from build123d import *


with BuildPart() as part:
    # BodySke → BaseBody (revolve)
    with BuildSketch(Plane.XY, mode=Mode.PRIVATE) as basebody_sk:
        with BuildLine():
            Line((21.808290377, 3.6), (25.5, 3.6))
            Line((25.5, 3.6), (25.5, 4))
            Line((25.5, 4), (28.472135955, 4))
            ThreePointArc((28.472135955, 4), (29.605034154, 2.140932539), (30, 0))
            Line((30, 0), (0, 0))
            Line((0, 0), (0, 4.172))
            Line((0, 4.172), (0.828, 5))
            Line((0.828, 5), (21, 5))
            Line((21, 5), (21.808290377, 3.6))
        make_face()
    revolve(basebody_sk.sketch.rotate(Axis((-3.175, 0, 0), (1, 0, 0)), 90), axis=Axis((-3.175, 0, 0), (1, 0, 0)))


solid = part.part
Verification items for the finished model (mm, model axes). Coordinates: 2 decimals unless noted, no trailing zeros. Order: outer loops, then holes, each group sorted by start corner. A loop starts at its lowest first (then second) coordinate and runs counter-clockwise, first axis right, second up. Notation, with made-up numbers: M -34,-18 L 13,-18 A19 cw 13,17 Z; hole C 33,29 d4. An arc over 180 degrees is marked long. One line per item, written item: value. Start each with the question number.
Item 1: Sectioned sample at A-A (y = 0). Enter the section's corners in (x, z).
Item 2: Gauge pin test, flat ends, axial feed: pin 1 (3 mm diameter, centred on x = 18.5, z = -3.5, fed in from +Y); pin 2 (1 mm diameter, centred on x = 18.5, z = -3, fed in from +Y); pin 3 (5 mm diameter, centred on x = 25, z = 0, fed in from -Y). Record the tip position at first contact, or that the pin passes through.
Item 3: Mould release check, pull along X, two halves, no side actions. Record for faces 1 (the flat face through (0, 0, 0)), 2 (the cylindrical face through (23.68, -1.081, 3.434)), 3 (the cylindrical face through (11, 0, -5)): released by +X, released by -X, zero draft, split by the parting line, or undercut.
Item 4: Sectioned sample at C-C (x = 4.5). Enter the section's corners in (y, z).
Item 5: Scan lines: probe 1 along Z at (x, y) = (6.5, 3); probe 2 along X at (y, z) = (-0.5, -3.75). Record each from-to range of solid material in increasing order.
Conclusion:
1. outline: M 0,-4.17 L 0.83,-5 L 21,-5 L 21.81,-3.6 L 25.5,-3.6 L 25.5,-4 L 28.47,-4 A6 ccw 28.47,4 L 25.5,4 L 25.5,3.6 L 21.81,3.6 L 21,5 L 0.83,5 L 0,4.17 Z
2. pin 1: stops at y = 4.58
2. pin 2: stops at y = 4.33
2. pin 3: stops at y = -4
3. face 1: released by -X
3. face 2: undercut
3. face 3: zero draft
4. outline: C 0,0 d10
5. probe 1: z = -4 to 4
5. probe 2: x = 0 to 21.7, 25.5 to 28.66
